For this review, take the finished solid that the model builds, in its own axes (mm). A direction names the side the tool comes from. Round coordinates to 2 decimals unless told otherwise and drop trailing zeros. Order: outer loops, then holes, each group sorted by start corner. A loop starts at its lowest first (then second) coordinate and runs counter-clockwise, first axis right, second up. Notation, with made-up numbers: M 35.5,62.25 L 81.5,62.25 A23 ccw 81.5,81.25 Z; hole C 74.5,31 d8. An arc over 180 degrees is marked long. Answer as a JSON object with one key per item and string values.
from build123d import *

# Parameters (mm, degrees)
SKETCH1_R           = 27.5
BOSS_EXTRUDE1_DEPTH = 1.5875
SKETCH4_R           = 3.55
SKETCH4_R_2         = 11.90625
CUT_EXTRUDE2_DEPTH  = 39.923259836
CUT_EXTRUDE1_DEPTH  = 0.79375


with BuildPart() as part:
    # Sketch1 → Boss-Extrude1 (new body)
    with BuildSketch(Plane(origin=(0, 0, 0), x_dir=(1, 0, 0), z_dir=(0, 1, 0))):
        with Locations(Location((0, 0, 0), (0, 0, 270))):
            Circle(SKETCH1_R)
    extrude(amount=BOSS_EXTRUDE1_DEPTH)

    # Sketch4 → Cut-Extrude2 (cut, through all)
    with BuildSketch(Plane.XZ):
        with Locations(Location((-20.0025, 0, 0), (0, 0, 270))):
            Circle(SKETCH4_R)
        with Locations(Location((0, 0, 0), (0, 0, 270))):
            Circle(SKETCH4_R_2)
        with Locations(Location((20.0025, 0, 0), (0, 0, 270))):
            Circle(SKETCH4_R)
    extrude(amount=-CUT_EXTRUDE2_DEPTH, mode=Mode.SUBTRACT)

    # Sketch2 → Cut-Extrude1 (cut)
    with BuildSketch(Plane(origin=(0, 1.5875, 0), x_dir=(1, 0, 0), z_dir=(0, 1, 0))):
        Polygon((0.302631579, -16.697368421), (-1.578947368, -16.697368421), (-1.578947368, -22), (-3.032894737, -22), (-3.032894737, -16.697368421), (-4.828947368, -16.697368421), (-4.828947368, -15.5), (0.302631579, -15.5), align=None)
        with BuildLine():
            Line((0.815789474, -21.72604852), (0.815789474, -20.289473684))
            add(Edge.make_bspline(
                [(0.815789474, -20.289473684), (0.882551721, -20.344188934), (1.014523687, -20.452347051), (1.227140713, -20.591115516), (1.447202728, -20.71001818), (1.675409001, -20.805403848), (1.908305656, -20.880763679), (2.143159037, -20.933694233), (2.379219718, -20.967619991), (2.536893399, -20.971660738), (2.615851151, -20.973684211)],
                knots=[0, 0, 0, 0, 1.052804814, 2.08112707, 3.092934838, 4.101597725, 5.095309197, 6.076510114, 7.036780032, 8, 8, 8, 8], degree=3))
            add(Edge.make_bspline(
                [(2.615851151, -20.973684211), (2.66087259, -20.973477518), (2.747938401, -20.9730778), (2.873639842, -20.961370885), (2.99073314, -20.94618485), (3.099082786, -20.923092555), (3.199279135, -20.895566542), (3.290917674, -20.86202374), (3.37356266, -20.823444156), (3.448177848, -20.780561289), (3.513594969, -20.732584572), (3.570415866, -20.680375528), (3.617618767, -20.623446094), (3.669442478, -20.543663794), (3.713452108, -20.432106591), (3.720266055, -20.338011829), (3.723684211, -20.290810033)],
                knots=[0, 0, 0, 0, 1.302764252, 2.519382516, 3.651968008, 4.719312502, 5.723721354, 6.658045591, 7.540747622, 8.361350842, 9.145473591, 9.884614119, 10.589667965, 11.280062621, 12.635567738, 14, 14, 14, 14], degree=3))
            add(Edge.make_bspline(
                [(3.723684211, -20.290810033), (3.722426598, -20.25997207), (3.719956321, -20.199398327), (3.69958044, -20.111022196), (3.664000491, -20.028974033), (3.616091236, -19.951631438), (3.556666419, -19.878233023), (3.487201128, -19.807648429), (3.407444856, -19.74029614), (3.284273886, -19.653302777), (3.10732717, -19.54775519), (2.867024513, -19.432171656), (2.601198691, -19.31429187), (2.415131632, -19.237352446), (2.319181743, -19.197676809)],
                knots=[0, 0, 0, 0, 0.590934481, 1.160748317, 1.727158715, 2.298507061, 2.900148301, 3.534378593, 4.194980596, 4.898998642, 6.423979724, 8.139194984, 10.009084388, 12, 12, 12, 12], degree=3))
            add(Edge.make_bspline(
                [(2.319181743, -19.197676809), (2.25788199, -19.17109541), (2.13808586, -19.119148238), (1.966708906, -19.032893283), (1.806493367, -18.944235596), (1.658517988, -18.850434485), (1.523442829, -18.751509678), (1.400085763, -18.64808955), (1.287457443, -18.541920664), (1.187708549, -18.43018436), (1.1001457, -18.312988169), (1.023877944, -18.190158763), (0.959369951, -18.061355383), (0.907178809, -17.926536043), (0.86553669, -17.786288337), (0.836246584, -17.639602069), (0.818473996, -17.487149218), (0.816692804, -17.383409336), (0.815789474, -17.330797697)],
                knots=[0, 0, 0, 0, 1.250860862, 2.444517047, 3.590871071, 4.678394788, 5.722744029, 6.723411862, 7.690959296, 8.618453783, 9.5242799, 10.426990097, 11.322232235, 12.217513229, 13.130682761, 14.058177248, 15.015205389, 16, 16, 16, 16], degree=3))
            add(Edge.make_bspline(
                [(0.815789474, -17.330797697), (0.818445505, -17.24958618), (0.823597707, -17.092051084), (0.860733455, -16.864521582), (0.924971912, -16.654859183), (1.016007936, -16.463914802), (1.126913051, -16.288854456), (1.259943872, -16.132191858), (1.408209222, -15.98883825), (1.57720384, -15.865185708), (1.760454764, -15.755197728), (1.958989864, -15.661820169), (2.171218494, -15.584552959), (2.396012169, -15.521863248), (2.631175245, -15.474928872), (2.874286713, -15.44009323), (3.123695328, -15.417908638), (3.292442744, -15.415625465), (3.377569901, -15.414473684)],
                knots=[0, 0, 0, 0, 1.081198718, 2.097322509, 3.059813659, 3.991166944, 4.906054364, 5.811353855, 6.721769168, 7.6459357, 8.59302305, 9.564157515, 10.562518314, 11.597307653, 12.668715501, 13.753374479, 14.866656162, 16, 16, 16, 16], degree=3))
            add(Edge.make_bspline(
                [(3.377569901, -15.414473684), (3.459987869, -15.415328313), (3.619994963, -15.416987499), (3.853159002, -15.427349754), (4.071558284, -15.446058754), (4.277161442, -15.471317206), (4.471658491, -15.504592658), (4.657344536, -15.546621391), (4.836054655, -15.593272055), (4.950256153, -15.633727811), (5.006578947, -15.653680099)],
                knots=[0, 0, 0, 0, 1.195237994, 2.320447403, 3.383723621, 4.373269299, 5.323774543, 6.243759987, 7.133843727, 8, 8, 8, 8], degree=3))
            Line((5.006578947, -15.653680099), (5.006578947, -16.953947368))
            add(Edge.make_bspline(
                [(5.006578947, -16.953947368), (4.950172841, -16.919417089), (4.834918543, -16.848861552), (4.648222275, -16.763029921), (4.452438329, -16.687693178), (4.250017568, -16.628897123), (4.045825372, -16.581321754), (3.843357111, -16.55035981), (3.646561557, -16.530718962), (3.517929378, -16.527761058), (3.455078125, -16.526315789)],
                knots=[0, 0, 0, 0, 0.973185875, 1.988505531, 3.020409709, 4.060289755, 5.089876897, 6.105810916, 7.074476093, 8, 8, 8, 8], degree=3))
            add(Edge.make_bspline(
                [(3.455078125, -16.526315789), (3.375169145, -16.528271218), (3.221521244, -16.53203109), (3.004767156, -16.569942483), (2.814066446, -16.626970822), (2.653815081, -16.70701684), (2.524891785, -16.806893537), (2.443308815, -16.906260816), (2.397741766, -16.993326378), (2.373865074, -17.061787316), (2.358331899, -17.134114289), (2.356304358, -17.183717359), (2.355263158, -17.209189967)],
                knots=[0, 0, 0, 0, 1.666493883, 3.204311803, 4.577720999, 5.808610471, 6.920989002, 7.959277989, 8.462502887, 8.965384053, 9.468694847, 10, 10, 10, 10], degree=3))
            add(Edge.make_bspline(
                [(2.355263158, -17.209189967), (2.356264289, -17.235551094), (2.358234991, -17.287442354), (2.374567326, -17.362801103), (2.402045011, -17.433762827), (2.453383319, -17.525132191), (2.547217166, -17.631338354), (2.688292429, -17.751715683), (2.86713992, -17.86247441), (3.075942128, -17.975041667), (3.317681453, -18.084059425), (3.489213426, -18.15617833), (3.579358553, -18.194078947)],
                knots=[0, 0, 0, 0, 0.477042346, 0.939046667, 1.388484856, 1.850770801, 2.82993316, 3.934162149, 5.200672571, 6.629956823, 8.228942609, 10, 10, 10, 10], degree=3))
            add(Edge.make_bspline(
                [(3.579358553, -18.194078947), (3.642418803, -18.220695676), (3.766433485, -18.273040301), (3.944706675, -18.359594534), (4.115266372, -18.44514729), (4.274023112, -18.537137812), (4.424922951, -18.629163804), (4.562535728, -18.730337502), (4.690337429, -18.835876907), (4.807037692, -18.948012462), (4.911345614, -19.067543538), (5.005777242, -19.193316325), (5.081813941, -19.330644509), (5.148791414, -19.474746561), (5.201449594, -19.629060676), (5.236481483, -19.79555739), (5.260393083, -19.973400477), (5.26221865, -20.096509128), (5.263157895, -20.159847862)],
                knots=[0, 0, 0, 0, 1.182142093, 2.324808002, 3.422600261, 4.4772321, 5.493523657, 6.473934373, 7.424665926, 8.355223432, 9.265842699, 10.163099642, 11.065981044, 11.971547163, 12.905946225, 13.874936649, 14.906666431, 16, 16, 16, 16], degree=3))
            add(Edge.make_bspline(
                [(5.263157895, -20.159847862), (5.260698876, -20.246423805), (5.255956928, -20.413376037), (5.21684268, -20.652638228), (5.153319213, -20.871196294), (5.061633909, -21.067198456), (4.947311835, -21.243154326), (4.81499893, -21.401271052), (4.663257063, -21.541638016), (4.494440069, -21.664634165), (4.308811924, -21.770101447), (4.109066808, -21.859488309), (3.894942021, -21.933562285), (3.667444469, -21.989651833), (3.429313461, -22.03179399), (3.183972553, -22.06221662), (2.931981847, -22.081521047), (2.761993293, -22.084180669), (2.675986842, -22.085526316)],
                knots=[0, 0, 0, 0, 1.135948082, 2.190551571, 3.17297232, 4.114787176, 5.019868708, 5.920575964, 6.814327848, 7.726634493, 8.65648264, 9.611815768, 10.59564518, 11.626721736, 12.684287895, 13.768626863, 14.871027011, 16, 16, 16, 16], degree=3))
            add(Edge.make_bspline(
                [(2.675986842, -22.085526316), (2.5873109, -22.084656233), (2.412455192, -22.08294056), (2.153423566, -22.064606065), (1.901063457, -22.036772954), (1.656381842, -21.999013651), (1.423487146, -21.948401798), (1.205239595, -21.887748169), (1.003210107, -21.814418992), (0.877301726, -21.755052086), (0.815789474, -21.72604852)],
                knots=[0, 0, 0, 0, 1.113719809, 2.196089038, 3.260137412, 4.302409517, 5.30443291, 6.252114794, 7.146074671, 8, 8, 8, 8], degree=3))
        make_face()
    extrude(amount=-CUT_EXTRUDE1_DEPTH, mode=Mode.SUBTRACT)


solid = part.part
1) Add section D-D on z = -16.5. State the section outline as (x, y) points.
Geometry check:
{"outline": "M -22,0 L 22,0 L 22,1.59 L -22,1.59 Z"}
2) Add section B-B on x = -8. State the section outline as (y, z) points.
Geometry check:
{"outline": "M 0,-26.31 L 1.59,-26.31 L 1.59,-8.82 L 0,-8.82 Z; M 0,8.82 L 1.59,8.82 L 1.59,26.31 L 0,26.31 Z"}
3) Insertion check: P1, Ø4, axis at x = -2, z = 19, coming from the +Y side; P2, Ø0.9, axis at y = 1.5, z = 16, coming from the -X side; P3, Ø0.6, axis at x = -4.5, y = 1.5, coming from the -Z side; P4, Ø19, axis at x = 0, z = 0, coming from the +Y side. Each pin has a flat end and moves straight along its axis. Give the tip position at first contact, or say it passes through.
Geometry check:
{"P1": "stops at y = 1.59", "P2": "stops at x = -22.68", "P3": "stops at z = -27.18", "P4": "passes through"}
4) For L1, parallel to X at y = 0.4, z = 0; L2, parallel to Z at x = 3, y = 1.3; L3, parallel to X at y = 0.3, z = 9, list the stretches that pass through material, from the lowest coordinate up.
Geometry check:
{"L1": "x = -27.5 to -23.55, -16.45 to -11.91, 11.91 to 16.45, 23.55 to 27.5", "L2": "z = -27.34 to -11.52, 11.52 to 15.43, 16.58 to 17.93, 19.5 to 20.94, 22.08 to 27.34", "L3": "x = -25.99 to -7.79, 7.79 to 25.99"}
5) Mouldability with a two-part tool opening along X and no side actions: class faces 1 (the cylindrical face through (-11.623, 0.783, 2.581)), 2 (the flat face through (-6, 1.588, 12)), 3 (the cylindrical face through (-24.397, 0.783, 12.69)) as +X half, -X half, draft (parallel to the pull), parting line (faces both ways), or undercut.
Geometry check:
{"face 1": "undercut", "face 2": "draft", "face 3": "parting line"}
6) Machinability: for faces 4 (the flat face through (-6, 0, 12)), 5 (the flat face through (3, 0.794, 19)), which of the approach directions +Z, -Z, +X, -X, +Y, -Y give a long, thin tool a straight path to every point of the face, cutting with its end or side? Answer none if there is none.
Geometry check:
{"face 4": "+Z, -Z, +X, -X, -Y", "face 5": "+Y"}
7) Add section A-A on z = 0. State the section outline as (x, y) points, and give its area (3 significant figures).
Geometry check:
{"outline": "M -27.5,0 L -23.55,0 L -23.55,1.59 L -27.5,1.59 Z; M -16.45,0 L -11.91,0 L -11.91,1.59 L -16.45,1.59 Z; M 11.91,0 L 16.45,0 L 16.45,1.59 L 11.91,1.59 Z; M 23.55,0 L 27.5,0 L 27.5,1.59 L 23.55,1.59 Z", "area": "27.0 mm²"}
8) Add section C-C on x = -18. State the section outline as (y, z) points.
Geometry check:
{"outline": "M 0,-20.79 L 1.59,-20.79 L 1.59,-2.93 L 0,-2.93 Z; M 0,2.93 L 1.59,2.93 L 1.59,20.79 L 0,20.79 Z"}
